Source: CAD feature listing. Evaluate the final solid. Frame: model axes, mm. A direction names the side the tool comes from. Round coordinates to 2 decimals unless told otherwise and drop trailing zeros. Order: outer loops, then holes, each group sorted by start corner. A loop starts at its lowest first (then second) coordinate and runs counter-clockwise, first axis right, second up.
Autodesk Inventor part; units mm, degrees
ref_plane "YZ Plane" through (0, 0, 0) normal (1, 0, 0) x (0, 1, 0)
ref_plane "XZ Plane" through (0, 0, 0) normal (0, 1, 0) x (-1, 0, 0)
ref_plane "XY Plane" through (0, 0, 0) normal (0, 0, 1) x (1, 0, 0)
sketch "Sketch1" plane through (0, 0, 0) normal (0, 1, 0) x (-1, 0, 0)
  line L0 (-6.395, -10.74) -> (6.395, -10.74)
  line L1 (6.395, -10.74) -> (8.355, -8.78)
  line L2 (8.355, -8.78) -> (8.355, 0.28)
  line L3 (8.355, 0.28) -> (5.235, 3.4)
  line L4 (5.235, 3.4) -> (5.235, 8.84)
  line L5 (5.235, 8.84) -> (4.07, 10.74)
  line L6 (-6.395, -10.74) -> (-8.355, -8.78)
  line L7 (-8.355, -8.78) -> (-8.355, 0.28)
  line L8 (-8.355, 0.28) -> (-5.235, 3.4)
  line L9 (-5.235, 3.4) -> (-5.235, 8.84)
  line L10 (-5.235, 8.84) -> (-4.07, 10.74)
  line L11 (-4.07, 10.74) -> (4.07, 10.74)
  dimension "d0" = 12.79
extrude "Extrusion1" add sketch "Sketch1" along normal blind 0.76
sketch "Sketch2" plane through (0, 0.76, 0) normal (0, 1, 0) x (1, 0, 0)
  line L0 (-5.235, -3.4) -> (5.235, -3.4) construction
  line L1 (5.235, -3.4) -> (5.235, -8.84) construction
  line L2 (5.235, -8.84) -> (-5.235, -8.84) construction
  line L3 (-5.235, -8.84) -> (-5.235, -3.4) construction
  line L4 (4.235, -4.4) -> (-4.235, -4.4)
  line L5 (-4.235, -4.4) -> (-4.235, -7.84)
  line L6 (-4.235, -7.84) -> (4.235, -7.84)
  line L7 (4.235, -7.84) -> (4.235, -4.4)
  point P0 (0, 0)
  dimension "d4" = 1
extrude "Extrusion2" add sketch "Sketch2" along normal blind 0.9
sketch "Sketch3" plane through (0, 0, 0) normal (0, -1, 0) x (1, 0, 0)
  line L0 (4.235, 4.4) -> (-4.235, 4.4)
  line L1 (-4.235, 4.4) -> (-4.235, 7.84)
  line L2 (-4.235, 7.84) -> (4.235, 7.84)
  line L3 (4.235, 7.84) -> (4.235, 4.4)
  point P0 (0, 0)
extrude "Extrusion3" add sketch "Sketch3" along normal blind 0.9
properties part number "WirebondAdapter"
1. Section D-D on z = -4. Return loops of the section in (x, y) (3 decimals), plus the area to 3 significant figures.
2. Section A-A on z = 6. Return loops of the section in (x, y) (3 decimals), plus the area to 3 significant figures.
3. Line query: line 1 along Y through (x, z) = (-3.25, 2.75); line 2 along Z through (x, y) = (-0.5, 1.2); line 3 along X through (y, z) = (0.2, 4.5) (3 decimals). Output: solid intervals per line, ascending.
4. First-contact query: pin 1 (1 mm diameter, centred on y = 1, z = 5.5, fed in from +X) (3 decimals); pin 2 (6 mm diameter, centred on x = -2.5, z = -2.5, fed in from +Y); pin 3 (0.6 mm diameter, centred on y = 0.5, z = 7, fed in from -X) (3 decimals). Flat tips, straight axial feed; report the tip coordinate or a pass-through.
5. Section C-C on y = 1. Return loops of the section in (x, z) (3 decimals).
6. Section B-B on x = 0.25. Return loops of the section in (y, z), plus the area to 3 significant figures.
7. Access query for faces 1 (the face through (0, 1, 7.84)), 2 (the face through (-0.1, -0.4, 7.84)), 3 (the face through (-4.235, -0.4, 6.1)). Directions: +Z, -Z, +X, -X, +Y, -Y. A direction counts if a zero-diameter tool reaches every point of the face in a straight line with its end or side. Return the directions, or none.
Result:
1. outline: (-8.355, 0) - (8.355, 0) - (8.355, 0.76) - (-8.355, 0.76) - close
1. area: 12.7 mm2
2. outline: (-5.235, 0) - (-4.235, 0) - (-4.235, -0.9) - (4.235, -0.9) - (4.235, 0) - (5.235, 0) - (5.235, 0.76) - (4.235, 0.76) - (4.235, 1.66) - (-4.235, 1.66) - (-4.235, 0.76) - (-5.235, 0.76) - close
2. area: 23.2 mm2
3. line 1: y = 0 to 0.76
3. line 2: z = 4.4 to 7.84
3. line 3: x = -5.235 to 5.235
4. pin 1: stops at x = 5.235
4. pin 2: stops at y = 0.76
4. pin 3: stops at x = -5.235
5. outline: (-4.235, 4.4) - (4.235, 4.4) - (4.235, 7.84) - (-4.235, 7.84) - close
6. outline: (-0.9, 4.4) - (0, 4.4) - (0, -10.74) - (0.76, -10.74) - (0.76, 4.4) - (1.66, 4.4) - (1.66, 7.84) - (0.76, 7.84) - (0.76, 10.74) - (0, 10.74) - (0, 7.84) - (-0.9, 7.84) - close
6. area: 22.5 mm2
7. face 1: +Z, +X, -X, +Y
7. face 2: +Z, +X, -X, -Y
7. face 3: +Z, -Z, -X, -Y
